The listing builds one solid part. Answer for the finished solid, in the listing's coordinates (mm). A direction names the side the tool comes from. Coordinates: 2 decimals unless noted, no trailing zeros. Write each loop counter-clockwise with the first axis right and the second up, starting at its lowest first coordinate (ties: lowest second). Pieces come first, ordered by that corner, then holes.
(1) The part is cut by section C-C on x = -13.5. Determine the outline of the cut face in (y, z).
(2) For a pull along X with two mould halves and no side action, classify faces 4 (the flat face through (-12, 7, 2)), 5 (the flat face through (-30, 6, 7)), 6 (the flat face through (-27, 7, 15)) as +X half, -X half, draft (parallel to the pull), parting line (faces both ways), or undercut.
(3) The part is cut by section A-A on y = 2.5. Determine the outline of the cut face in (x, z), plus the area to 3 significant figures.
(4) Given P1, Ø2, axis at x = -1, y = 2.5, coming from the -Z side; P2, Ø3, axis at x = 2.5, y = 5.5, coming from the +Z side; P3, Ø4, axis at x = -12, y = 4, coming from the +Z side, each flat-ended and moving along its own axis, determine where each tip first touches the part or whether it passes through.
(5) Straight lines are drawn through the part: line 1 (X direction, y = 6.5, z = 4); line 2 (X direction, y = 6.5, z = 10.25); line 3 (Z direction, x = -17.5, y = 6.25). For each, find the intervals that lie inside material, in ascending order.
(6) Which of the six approach directions +Z, -Z, +X, -X, +Y, -Y give full straight-line access (tool end or side, diameter ignored) to faces 1 (the flat face through (-13, 7, 0)), 2 (the flat face through (2, 7, 5.5)), 3 (the flat face through (0, 6, 4))?
(7) The part is cut by section B-B on z = 7.5. Determine the outline of the cut face in (x, y).
from build123d import *

# Parameters (mm, degrees)
F0_W     = 7
F0_H     = 13.09483
F1_DEPTH = 15
F0_W_2   = 23
F2_DEPTH = 2
F0_W_3   = 4
F3_DEPTH = 5.5


with BuildPart() as f1:
    # F0 (on Top) → F1 (new body)
    with BuildSketch(Plane.XY):
        with Locations((-26.5, 6.547415)):
            Rectangle(F0_W, F0_H)
    extrude(amount=F1_DEPTH)

    # F0 (on Top) → F2 (join)
    with BuildSketch(Plane.XY):
        with Locations((-11.5, 6.547415)):
            Rectangle(F0_W_2, F0_H)
    extrude(amount=F2_DEPTH)

    # F0 (on Top) → F3 (join)
    with BuildSketch(Plane.XY):
        with Locations((2, 6.547415)):
            Rectangle(F0_W_3, F0_H)
    extrude(amount=F3_DEPTH)


solid = f1.part
Model answer:
1. outline: (0, 0) - (13.09, 0) - (13.09, 2) - (0, 2) - close
2. face 4: undercut
2. face 5: -X half
2. face 6: draft
3. outline: (-30, 0) - (4, 0) - (4, 5.5) - (0, 5.5) - (0, 2) - (-23, 2) - (-23, 15) - (-30, 15) - close
3. area: 173 mm2
4. P1: stops at z = 0
4. P2: stops at z = 5.5
4. P3: stops at z = 2
5. line 1: x = -30 to -23, 0 to 4
5. line 2: x = -30 to -23
5. line 3: z = 0 to 2
6. face 1: -Z, +X, -X, +Y, -Y
6. face 2: +Z, +X, +Y, -Y
6. face 3: +Z, +Y, -Y
7. outline: (-30, 0) - (-23, 0) - (-23, 13.09) - (-30, 13.09) - close
